Input: part model. Units: mm. Frame: model coordinates. Round coordinates to 2 decimals unless told otherwise and drop trailing zeros. Write each loop counter-clockwise with the first axis right and the second up, starting at its lowest first coordinate (ties: lowest second). Pieces come first, ordered by that corner, then holes. Notation, with made-up numbers: (67.5, 37.25) - (98.5, 37.25) arc R14 cw to (98.5, 49.25) - close; hole circle Ø5 at (12, -9). An arc over 180 degrees is marked (long way). One line per item, written item: value. Start each with the question number.
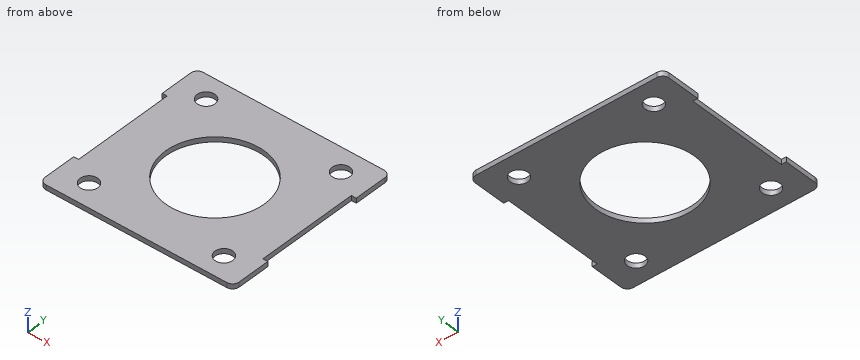
```python
from build123d import *

# Parameters (mm, degrees)
SKETCH1_W          = 187.325
SKETCH1_H          = 174.625
EXTRUDE1_DEPTH     = 4.7625
CUT_EXTRUDE1_REACH = 130.136
SKETCH2_W          = 4.7625
SKETCH2_H          = 98.425
FILLET1_R          = 6.35
CUT_EXTRUDE2_REACH = 130.136
SKETCH3_R          = 47.625
SKETCH3_R_2        = 8.5328125


with BuildPart() as part:
    # Sketch1 → Extrude1 (new body)
    with BuildSketch(Plane.XY):
        Rectangle(SKETCH1_W, SKETCH1_H)
    extrude(amount=EXTRUDE1_DEPTH)

    # Sketch2 → Cut-Extrude1 (cut, up to next)
    with BuildSketch(Plane.XY.offset(4.7625), mode=Mode.PRIVATE) as cut_extrude1_sk1:
        with Locations((-91.28125, 0)):
            Rectangle(SKETCH2_W, SKETCH2_H)
    cut_extrude1_tool1 = extrude(cut_extrude1_sk1.sketch, amount=-CUT_EXTRUDE1_REACH, mode=Mode.PRIVATE) & part.part
    # Sketch2 → Cut-Extrude1 (cut, up to next)
    with BuildSketch(Plane.XY.offset(4.7625), mode=Mode.PRIVATE) as cut_extrude1_sk2:
        with Locations((91.28125, 0)):
            Rectangle(SKETCH2_W, SKETCH2_H)
    cut_extrude1_tool2 = extrude(cut_extrude1_sk2.sketch, amount=-CUT_EXTRUDE1_REACH, mode=Mode.PRIVATE) & part.part
    add(cut_extrude1_tool1.solids().sort_by_distance((-91.28125, 0, 4.7625))[0], mode=Mode.SUBTRACT)
    add(cut_extrude1_tool2.solids().sort_by_distance((91.28125, 0, 4.7625))[0], mode=Mode.SUBTRACT)

    # Fillet1
    fillet1_edges = [part.edges().sort_by_distance(p)[0] for p in [
        (-93.6625, 87.3125, 2.38125),
        (93.6625, 87.3125, 2.38125),
        (93.6625, -87.3125, 2.38125),
        (-93.6625, -87.3125, 2.38125),
    ]]
    fillet(fillet1_edges, radius=FILLET1_R)

    # Sketch3 → Cut-Extrude2 (cut, up to next)
    with BuildSketch(Plane.XY.offset(4.7625), mode=Mode.PRIVATE) as cut_extrude2_sk1:
        Circle(SKETCH3_R)
    cut_extrude2_tool1 = extrude(cut_extrude2_sk1.sketch, amount=-CUT_EXTRUDE2_REACH, mode=Mode.PRIVATE) & part.part
    # Sketch3 → Cut-Extrude2 (cut, up to next)
    with BuildSketch(Plane.XY.offset(4.7625), mode=Mode.PRIVATE) as cut_extrude2_sk2:
        with Locations((-65.0875, 65.0875)):
            Circle(SKETCH3_R_2)
    cut_extrude2_tool2 = extrude(cut_extrude2_sk2.sketch, amount=-CUT_EXTRUDE2_REACH, mode=Mode.PRIVATE) & part.part
    # Sketch3 → Cut-Extrude2 (cut, up to next)
    with BuildSketch(Plane.XY.offset(4.7625), mode=Mode.PRIVATE) as cut_extrude2_sk3:
        with Locations((-65.0875, -65.0875)):
            Circle(SKETCH3_R_2)
    cut_extrude2_tool3 = extrude(cut_extrude2_sk3.sketch, amount=-CUT_EXTRUDE2_REACH, mode=Mode.PRIVATE) & part.part
    # Sketch3 → Cut-Extrude2 (cut, up to next)
    with BuildSketch(Plane.XY.offset(4.7625), mode=Mode.PRIVATE) as cut_extrude2_sk4:
        with Locations((65.0875, -65.0875)):
            Circle(SKETCH3_R_2)
    cut_extrude2_tool4 = extrude(cut_extrude2_sk4.sketch, amount=-CUT_EXTRUDE2_REACH, mode=Mode.PRIVATE) & part.part
    # Sketch3 → Cut-Extrude2 (cut, up to next)
    with BuildSketch(Plane.XY.offset(4.7625), mode=Mode.PRIVATE) as cut_extrude2_sk5:
        with Locations((65.0875, 65.0875)):
            Circle(SKETCH3_R_2)
    cut_extrude2_tool5 = extrude(cut_extrude2_sk5.sketch, amount=-CUT_EXTRUDE2_REACH, mode=Mode.PRIVATE) & part.part
    add(cut_extrude2_tool1.solids().sort_by_distance((0, 0, 4.7625))[0], mode=Mode.SUBTRACT)
    add(cut_extrude2_tool2.solids().sort_by_distance((-65.0875, 65.0875, 4.7625))[0], mode=Mode.SUBTRACT)
    add(cut_extrude2_tool3.solids().sort_by_distance((-65.0875, -65.0875, 4.7625))[0], mode=Mode.SUBTRACT)
    add(cut_extrude2_tool4.solids().sort_by_distance((65.0875, -65.0875, 4.7625))[0], mode=Mode.SUBTRACT)
    add(cut_extrude2_tool5.solids().sort_by_distance((65.0875, 65.0875, 4.7625))[0], mode=Mode.SUBTRACT)


solid = part.part
```
Q1. Contact query for flat-ended pins moving along their axis: pin 1 Ø13.5 at (x, y) = (65.09, 65.09) entering from -Z; pin 2 Ø1 at (y, z) = (-6, 3.5) entering from -X; pin 3 Ø1.4 at (x, z) = (-91.5, 2) entering from -Y; pin 4 Ø2.5 at (y, z) = (2, 3.5) entering from +X. Output: stop coordinate, or through.
Q2. Cut plane A-A, the plane y = 0. Output: boundary loops of the cut face in (x, z) (1 decimal).
Q3. Cut plane C-C, the plane x = -68. Output: boundary loops of the cut face in (y, z), and give its area (3 significant figures).
Q4. Cut plane B-B, the plane x = 0. Output: boundary loops of the cut face in (y, z) (1 decimal), and give its area (3 significant figures).
Q5. Material intervals for probe 1 along X at (y, z) = (-66, 4.2); probe 2 along X at (y, z) = (62, 1.35); probe 3 along X at (y, z) = (-3, 0.2), sorted ascending. Write a range as from..to.
Q6. Cut plane D-D, the plane z = 0.9. Count the separate pieces of the cut face and the enclosed holes in it, and give its area (3 significant figures).
A:
1. pin 1: passes through
1. pin 2: stops at x = -88.9
1. pin 3: stops at y = -86.27
1. pin 4: stops at x = 88.9
2. outline: (-88.9, 0) - (-47.6, 0) - (-47.6, 4.8) - (-88.9, 4.8) - close; (47.6, 0) - (88.9, 0) - (88.9, 4.8) - (47.6, 4.8) - close
3. outline: (-87.31, 0) - (-73.11, 0) - (-73.11, 4.76) - (-87.31, 4.76) - close; (-57.07, 0) - (57.07, 0) - (57.07, 4.76) - (-57.07, 4.76) - close; (73.11, 0) - (87.31, 0) - (87.31, 4.76) - (73.11, 4.76) - close
3. area: 679 mm²
4. outline: (-87.3, 0) - (-47.6, 0) - (-47.6, 4.8) - (-87.3, 4.8) - close; (47.6, 0) - (87.3, 0) - (87.3, 4.8) - (47.6, 4.8) - close
4. area: 378 mm²
5. probe 1: x = -93.66..-73.57, -56.6..56.6, 73.57..93.66
5. probe 2: x = -93.66..-73.04, -57.13..57.13, 73.04..93.66
5. probe 3: x = -88.9..-47.53, 47.53..88.9
6. separate pieces: 1
6. enclosed holes: 5
6. area: 23,700 mm²
